Input: part model. Units: mm. Frame: model coordinates. A direction names the side the tool comes from. Round coordinates to 2 decimals unless told otherwise and drop trailing zeros. Write each loop counter-clockwise with the first axis right and the second up, starting at its lowest first coordinate (ties: lowest second). Pieces come first, ordered by that corner, then holes. Notation, with made-up numbers: (18, 35) -> (52, 35) arc R15 ccw to (52, 55) -> close; hole circle Ø4 at (25.5, 72). An arc over 180 degrees is marked (long way). Use CSV: the item, a comma, the result in double quotes.
```python
from build123d import *

# Parameters (mm, degrees)
SKETCH_1_W          = 50
SKETCH_1_H          = 30
EXTRUDE_1_DEPTH     = 35
SKETCH_2_W          = 15
SKETCH_2_H          = 15
CUT_EXTRUDE_1_DEPTH = 46.552167896
SKETCH_3_W          = 13.5
SKETCH_3_H          = 10
CUT_EXTRUDE_2_DEPTH = 15
SKETCH_3_3_W        = 8
SKETCH_3_3_H        = 12.5
SKETCH_3_3_H_2      = 10
SKETCH_3_3_H_3      = 7.5
SKETCH_3_3_W_2      = 6.5
CUT_EXTRUDE_3_DEPTH = 7
SKETCH_6_W          = 5
SKETCH_6_H          = 13
CUT_EXTRUDE_4_DEPTH = 6
CUT_EXTRUDE_5_REACH = 54.44
SKETCH_7_W          = 13.5
SKETCH_7_H          = 17
CUT_EXTRUDE_6_DEPTH = 5
CUT_EXTRUDE_7_DEPTH = 5


with BuildPart() as part:
    # Эскиз1 → Бобышка-Вытянуть1 (new body)
    with BuildSketch(Plane.XY):
        Rectangle(SKETCH_1_W, SKETCH_1_H)
    extrude(amount=EXTRUDE_1_DEPTH)

    # Эскиз2 → Вырез-Вытянуть1 (cut, through all)
    with BuildSketch(Plane.XY.offset(35)):
        with Locations((17.5, 7.5)):
            Rectangle(SKETCH_2_W, SKETCH_2_H)
    extrude(amount=-CUT_EXTRUDE_1_DEPTH, mode=Mode.SUBTRACT)

    # Эскиз3 → Вырез-Вытянуть2 (cut)
    with BuildSketch(Plane(origin=(0, 15, 0), x_dir=(1, 0, 0), z_dir=(0, 1, 0))):
        with Locations((3.25, -17.5)):
            Rectangle(SKETCH_3_W, SKETCH_3_H)
    extrude(amount=-CUT_EXTRUDE_2_DEPTH, mode=Mode.SUBTRACT)

    # Эскиз3<3> → Вырез-Вытянуть3 (cut)
    with BuildSketch(Plane(origin=(0, 15, 0), x_dir=(1, 0, 0), z_dir=(0, 1, 0))):
        with Locations((-7.5, -28.75)):
            Rectangle(SKETCH_3_3_W, SKETCH_3_3_H)
        with Locations((-7.5, -17.5)):
            Rectangle(SKETCH_3_3_W, SKETCH_3_3_H_2)
        with Locations((-7.5, -8.75)):
            Rectangle(SKETCH_3_3_W, SKETCH_3_3_H_3)
        with Locations((-14.75, -17.5)):
            Rectangle(SKETCH_3_3_W_2, SKETCH_3_3_H_2)
    extrude(amount=-CUT_EXTRUDE_3_DEPTH, mode=Mode.SUBTRACT)

    # Эскиз6 → Вырез-Вытянуть4 (cut)
    with BuildSketch(Plane(origin=(0, 0, 0), x_dir=(1, 0, 0), z_dir=(0, 1, 0))):
        with Locations((22.5, -17.5)):
            Rectangle(SKETCH_6_W, SKETCH_6_H)
    extrude(amount=-CUT_EXTRUDE_4_DEPTH, mode=Mode.SUBTRACT)

    # Вырез-Вытянуть5: up to this face of the body (flat: up to its plane)
    cut_extrude_5_end = Plane(part.part.faces().sort_by_distance((13.720588235, 0, 17.5))[0])
    # Эскиз7 → Вырез-Вытянуть5 (cut, up to the picked face)
    with BuildSketch(Plane(origin=(0, 15, 0), x_dir=(1, 0, 0), z_dir=(0, 1, 0)), mode=Mode.PRIVATE) as cut_extrude_5_sk1:
        with Locations((3.25, -17.5)):
            Rectangle(SKETCH_7_W, SKETCH_7_H)
    cut_extrude_5_tool1 = split(extrude(cut_extrude_5_sk1.sketch, amount=-CUT_EXTRUDE_5_REACH, mode=Mode.PRIVATE), bisect_by=cut_extrude_5_end, keep=Keep.BOTH, mode=Mode.PRIVATE)
    add(cut_extrude_5_tool1.solids().sort_by(Axis((3.25, 15, 17.5), (0, -1, 0)))[0], mode=Mode.SUBTRACT)

    # Эскиз8 → Вырез-Вытянуть6 (cut)
    with BuildSketch(Plane.XY.offset(35)):
        with BuildLine():
            Line((25, 0), (10, 0))
            ThreePointArc((10, 0), (20.606601718, -4.393398282), (25, -15))
            Line((25, -15), (25, 0))
        make_face()
    extrude(amount=-CUT_EXTRUDE_6_DEPTH, mode=Mode.SUBTRACT)

    # Эскиз9 → Вырез-Вытянуть7 (cut)
    with BuildSketch(Plane(origin=(0, 0, 0), x_dir=(-1, 0, 0), z_dir=(0, 0, -1))):
        Polygon((-25, -15), (-10, 0), (-25, 0), align=None)
    extrude(amount=-CUT_EXTRUDE_7_DEPTH, mode=Mode.SUBTRACT)


solid = part.part
```
Item 1: Set-up query: faces 4 (the face through (-3.5, 12, 31)), 5 (the face through (20.49, -4.28, 32.53)), 6 (the face through (20, -3, 18)). Return all of +Z, -Z, +X, -X, +Y, -Y with unobstructed straight access to the full face (end or side cutting, diameter ignored); none if empty.
Worked answers:
face 4,"+Z, +Y"
face 5,"+Z, +X, +Y"
face 6,"+X, +Y"
Item 2: Section query C-C on z = 6. Return the cut outline in (x, y), plus the area to 3 significant figures.
Worked answers:
outline,"(-25, -15) -> (25, -15) -> (25, 0) -> (10, 0) -> (10, 15) -> (-3.5, 15) -> (-3.5, 8) -> (-11.5, 8) -> (-11.5, 15) -> (-25, 15) -> close"
area,"1,220 mm²"
Item 3: Line query: line 1 (Z direction, x = 21, y = -1.25); line 2 (X direction, y = 13.25, z = 8.5); line 3 (Z direction, x = 1, y = 13.75). Output: solid intervals per line, ascending.
Worked answers:
line 1,"z = 5 to 11, 24 to 30"
line 2,"x = -25 to -11.5, -3.5 to 10"
line 3,"z = 0 to 9, 26 to 35"
Item 4: Section query B-B on y = -8.75. Return the cut outline in (x, z).
Worked answers:
outline,"(-25, 0) -> (18.75, 0) -> (18.75, 5) -> (25, 5) -> (25, 30) -> (23.64, 30) -> (23.64, 35) -> (-25, 35) -> close"
Item 5: Section query D-D on x = -8.5. Return the cut outline in (y, z).
Worked answers:
outline,"(-15, 0) -> (15, 0) -> (15, 5) -> (8, 5) -> (8, 35) -> (-15, 35) -> close"
Item 6: Pull-direction query (X, two-part tool) for faces 1 (the face through (-25, 0, 17)), 2 (the face through (-3.5, 12, 7)), 3 (the face through (22, -6, 17)); classes: +X half, -X half, draft (parallel to the pull), parting line (faces both ways), or undercut.
Worked answers:
face 1,"-X half"
face 2,"undercut"
face 3,"draft"
Item 7: Section query A-A on x = -14.5. Return the cut outline in (y, z), plus the area to 3 significant figures.
Worked answers:
outline,"(-15, 0) -> (15, 0) -> (15, 12.5) -> (8, 12.5) -> (8, 22.5) -> (15, 22.5) -> (15, 35) -> (-15, 35) -> close"
area,"980 mm²"
Item 8: First-contact query: pin 1 Ø5 at (y, z) = (8.5, 21) entering from +X; pin 2 Ø3.5 at (y, z) = (11, 18.5) entering from +X; pin 3 Ø5.5 at (x, z) = (23, 16) entering from +Y. Flat tips, straight axial feed; report the tip coordinate or a pass-through.
Worked answers:
pin 1,"stops at x = -3.5"
pin 2,"stops at x = -18"
pin 3,"stops at y = -6"
